Design review of the part built by this model. Coordinates are the model's own, in mm. A direction names the side the tool comes from. Coordinates: 2 decimals unless noted, no trailing zeros. Write each loop counter-clockwise with the first axis right and the second up, starting at its lowest first coordinate (ties: lowest second). Pieces come first, ordered by that corner, then holes.
Q1. For L1, parallel to Y at x = 0, z = 23; L2, parallel to Z at x = -38, y = -26.5; L3, parallel to X at y = -30, z = 13.5, list the stretches that pass through material, from the lowest coordinate up.
Q2. For pin 1 Ø12 at (y, z) = (-30.5, 22) entering from -X; pin 2 Ø4 at (x, z) = (-26, 10) entering from -Y; pin 3 Ø12 at (x, z) = (15, 17) entering from -Y, all flat-tipped, find the tip position at first contact; note any pin that passes through.
Q3. Take a section at A-A, the plane x = 0. Write out the cut boundary in (y, z), plus the area to 3 significant figures.
Q4. Take a section at B-B, the plane z = 24.5. Write out the cut boundary in (x, y), plus the area to 3 significant figures.
Q5. Take a section at C-C, the plane y = -10.5. Write out the cut boundary in (x, z).
Q6. The part is to be moulded in two halves that separate along X. For faces 3 (the flat face through (-1, 1, 7.75)), 4 (the cylindrical face through (-53.428, 2.351, 3.821)), 5 (the flat face through (-1, 1, 0)), say which applies: released by +X, released by -X, zero draft, split by the parting line, or undercut.
Q7. For faces 1 (the flat face through (12, 40, 7.75)), 2 (the flat face through (-36.3, 12.2, 48.746)), list the 3-axis set-ups (+Z, -Z, +X, -X, +Y, -Y) from which the entire face can be reached by the end or side of a thin tool; tool diameter is ignored.
Q8. Take a section at D-D, the plane z = 5. Write out the cut boundary in (x, y).
from build123d import *

# Parameters (mm, degrees)
F0_R     = 40.671356
F1_DEPTH = 48.746474
F3_D     = 76.2
F4_R     = 53.479335
F5_DEPTH = 7.750219


with BuildPart() as f1:
    # F0 (on Top) → F1 (new body)
    with BuildSketch(Plane.XY):
        Circle(F0_R)
    extrude(amount=F1_DEPTH)

    # F3 (through all)
    with Locations(Plane.XY.offset(48.746474)):
        with Locations((0, 0)):
            Hole(F3_D / 2)

    # F4 (on Top) → F5 (join)
    with BuildSketch(Plane.XY):
        Circle(F4_R)
    extrude(amount=F5_DEPTH)


solid = f1.part
Responses:
1. L1: y = -40.67 to -38.1, 38.1 to 40.67
1. L2: z = 0 to 7.75
1. L3: x = -27.46 to -23.49, 23.49 to 27.46
2. pin 1: stops at x = -32.46
2. pin 2: stops at y = -32.84
2. pin 3: stops at y = -39.66
3. outline: (-53.48, 0) - (53.48, 0) - (53.48, 7.75) - (40.67, 7.75) - (40.67, 48.75) - (38.1, 48.75) - (38.1, 7.75) - (-38.1, 7.75) - (-38.1, 48.75) - (-40.67, 48.75) - (-40.67, 7.75) - (-53.48, 7.75) - close
3. area: 1,040 mm2
4. outline: circle Ø81.34 at (0, 0); hole circle Ø76.2 at (0, 0)
4. area: 636 mm2
5. outline: (-52.44, 0) - (52.44, 0) - (52.44, 7.75) - (39.29, 7.75) - (39.29, 48.75) - (36.62, 48.75) - (36.62, 7.75) - (-36.62, 7.75) - (-36.62, 48.75) - (-39.29, 48.75) - (-39.29, 7.75) - (-52.44, 7.75) - close
6. face 3: undercut
6. face 4: split by the parting line
6. face 5: zero draft
7. face 1: +Z
7. face 2: +Z, +X, -X, +Y, -Y
8. outline: circle Ø106.96 at (0, 0)
